Can you work these out from the model? Positions are in its coordinate system, mm. Coordinates: 2 decimals unless noted, no trailing zeros. Order: outer loops, then holes, each group sorted by start corner. A loop starts at its lowest first (then second) coordinate and runs counter-clockwise, first axis right, second up. Notation, with made-up numbers: (75.5, -8.75) - (113.5, -8.75) arc R20 ccw to (113.5, 10.25) - close; hole circle Ø2 at (-34, 41). An arc over 180 degrees is marked (long way). Return JSON: item names as keys, results as strings. Group by question number.
1) For pin 1 Ø2.5 at (x, y) = (9, 0) entering from -Z; pin 2 Ø5.5 at (x, z) = (9, -33.33) entering from -Y; pin 3 Ø2.5 at (x, z) = (7.5, 32.5) entering from +Y; pin 4 Ø10.5 at (x, z) = (9, 33.33) entering from -Y (3 decimals), each with a flat end and sliding along its axis, tell me the tip position at first contact or that it passes through.
2) Imagine slicing it at D-D (y = -15.5). Write out the boundary of the cut face in (x, z), and give its area (3 significant figures).
3) Imagine slicing it at B-B (y = 0). Write out the boundary of the cut face in (x, z).
4) If I drill on line 1 along Z through (x, y) = (9, 25.9); line 2 along Y through (x, z) = (9, 31.5); line 3 along Y through (x, z) = (8.75, 74.5), over which ranges is the centre line in solid material (lowest first)?
5) Imagine slicing it at C-C (z = 10.5). Write out the boundary of the cut face in (x, y), and give its area (3 significant figures).
6) Imagine slicing it at A-A (x = 9). Write out the boundary of the cut face in (y, z).
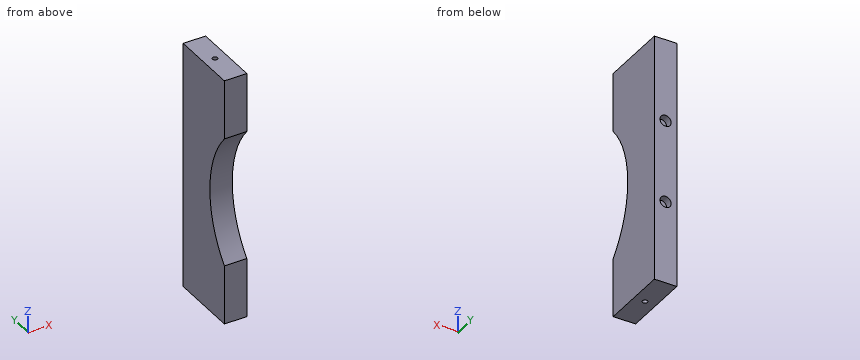
Autodesk Inventor part; units mm, degrees
ref_plane "YZ Plane" through (0, 0, 0) normal (1, 0, 0) x (0, 1, 0)
ref_plane "XZ Plane" through (0, 0, 0) normal (0, 1, 0) x (-1, 0, 0)
ref_plane "XY Plane" through (0, 0, 0) normal (0, 0, 1) x (1, 0, 0)
sketch "Boceto1" plane through (0, 0, 0) normal (1, 0, 0) x (0, 1, 0)
  line L0 (27.5, -100) -> (-27.5, -100)
  line L1 (-27.5, -100) -> (-27.5, 100)
  line L2 (-27.5, 100) -> (27.5, 100)
  line L3 (27.5, 100) -> (27.5, -100)
  line L4 (27.5, -100) -> (-27.5, 100) construction
  line L5 (-27.5, -100) -> (27.5, 100) construction
  point P0 (0, 0)
  dimension "alto" = 55
  dimension "ancho" = 200
extrude "Extrusión1" add sketch "Boceto1" along normal blind 18
sketch "Boceto2" plane through (0, 27.5, 100) normal (0, 1, 0) x (1, 0, 0)
  circle A0 centre (9, 66.6667) radius 4.5
  circle A1 centre (9, 133.3333) radius 4.5
  line L0 (0, 0) -> (18, 0)
  line L1 (0, 200) -> (18, 200)
  line L2 (18, 200) -> (18, 0)
  point P0 (0, 100)
  dimension "d4" = 9
  dimension "d5" = 9
  dimension "alto1" = 66.6667
  dimension "d7" = 66.6667
  dimension "d8" = 9
  dimension "d9" = 9
extrude "Extrusión2" cut sketch "Boceto2" against normal blind 6
sketch "Boceto3" plane through (18, 0, 0) normal (1, 0, 0) x (0, 0, -1)
  circle A0 centre (0, -88.1077) radius 80
  line L0 (-100, 27.5) -> (-100, -27.5)
  point P0 (0, 0)
  dimension "radio" = 160
  dimension "d14" = 100
extrude "Extrusión3" cut sketch "Boceto3" against normal blind 18
sketch "Boceto4" plane through (0, -27.5, 100) normal (0, 0, 1) x (1, 0, 0)
  circle A0 centre (9, 27.5) radius 2
  line L0 (0, 55) -> (18, 55)
  point P0 (0, 27.5)
  point P1 (9, 55)
  dimension "d17" = 4
  dimension "d18" = 27.5
extrude "Extrusión4" cut sketch "Boceto4" against normal blind 290
equation "\"d4\" = 0.5 * grosor"
equation "\"d5\" = d4"
equation "\"d7\" = alto1"
equation "\"d8\" = d9"
equation "\"d9\" = 0.5 * grosor"
equation "\"d10\" = 0.333333 * grosor"
equation "\"d14\" = 0.5 * ancho"
equation "\"d15\" = grosor"
properties part number "APM_003-1"
Calculated:
{
 "1": {"pin 1": "through", "pin 2": "y = -16.71", "pin 3": "y = 21.5", "pin 4": "y = -18.025"},
 "2": {"outline": "(0, -100) - (18, -100) - (18, -33.59) - (0, -33.59) - close; (0, 33.59) - (18, 33.59) - (18, 100) - (0, 100) - close", "area": "2,390 mm2"},
 "3": {"outline": "(0, -100) - (7, -100) - (7, 100) - (0, 100) - close; (11, -100) - (18, -100) - (18, 100) - (11, 100) - close"},
 "4": {"line 1": "-100 to -37.83, -28.83 to 28.83, 37.83 to 100", "line 2": "-14.57 to -2, 2 to 21.5", "line 3": "-27.5 to -1.98, 1.98 to 27.5"},
 "5": {"outline": "(0, -8.8) - (18, -8.8) - (18, 27.5) - (0, 27.5) - close; hole circle Ø4 at (9, 0)", "area": "641 mm2"},
 "6": {"outline": "(-27.5, -100) - (-2, -100) - (-2, 100) - (-27.5, 100) - (-27.5, 52.22) arc R80 cw to (-27.5, -52.22) - close; (2, -100) - (27.5, -100) - (27.5, -37.83) - (21.5, -37.83) - (21.5, -28.83) - (27.5, -28.83) - (27.5, 28.83) - (21.5, 28.83) - (21.5, 37.83) - (27.5, 37.83) - (27.5, 100) - (2, 100) - close"}
}
